Verification items for this drawing (mm, ordinates from the low corner). A direction names the side the tool comes from. Round coordinates to 2 decimals unless told otherwise and drop trailing zeros. Loops run counter-clockwise (first coordinate to the right, second up) from the corner with the lowest first, then second, coordinate; pieces in that order, holes last. Notation, with made-up numbers: M 35,67.25 L 66,67.25 A7 cw 66,75.25 Z; hole C 5,71 d9. An arc over 180 degrees is marked long. Write item = value, one per line. Start each with the question number.
(1) Cross-section at A-A on x = 21.5. Record the boundary of the cut face in (y, z), plus the area to 3 significant figures.
(2) Cross-section at D-D on x = 12. Record the boundary of the cut face in (y, z), plus the area to 3 significant figures.
(3) Mould release check, pull along Y, two halves, no side actions. Record for the marked faces 5, 6, 7 and 8: pulls with the +Y half, pulls with the -Y half, needs draft (parallel to the pull), parting line crosses it, or undercut.
(4) Set-up check for the marked faces 1, 2, 3 and 4: record each of +Z, -Z, +X, -X, +Y, -Y from which the full face is reachable in a straight line by a thin tool's end or side.
(5) Cross-section at B-B on y = 27.6. Record the boundary of the cut face in (x, z).
(6) Scan lines: L1, parallel to Y at x = 21.5, z = 6.5; L2, parallel to X at y = 27.5, z = 5; L3, parallel to Z at x = 8.5, y = 14.5. Record each from-to range of solid material in increasing order. Write a range as from..to.
(7) Cross-section at C-C on y = 5. Record the boundary of the cut face in (x, z).
(8) Go/stop test with flat-tipped pins: P1, Ø16, axis at x = 15.5, z = 21.5, coming from the +Y side; P2, Ø5, axis at y = 2.5, z = 14.5, coming from the -X side; P3, Ø11, axis at y = 5.5, z = 20.5, coming from the +X side. Record where each tip stops, or that it passes through.
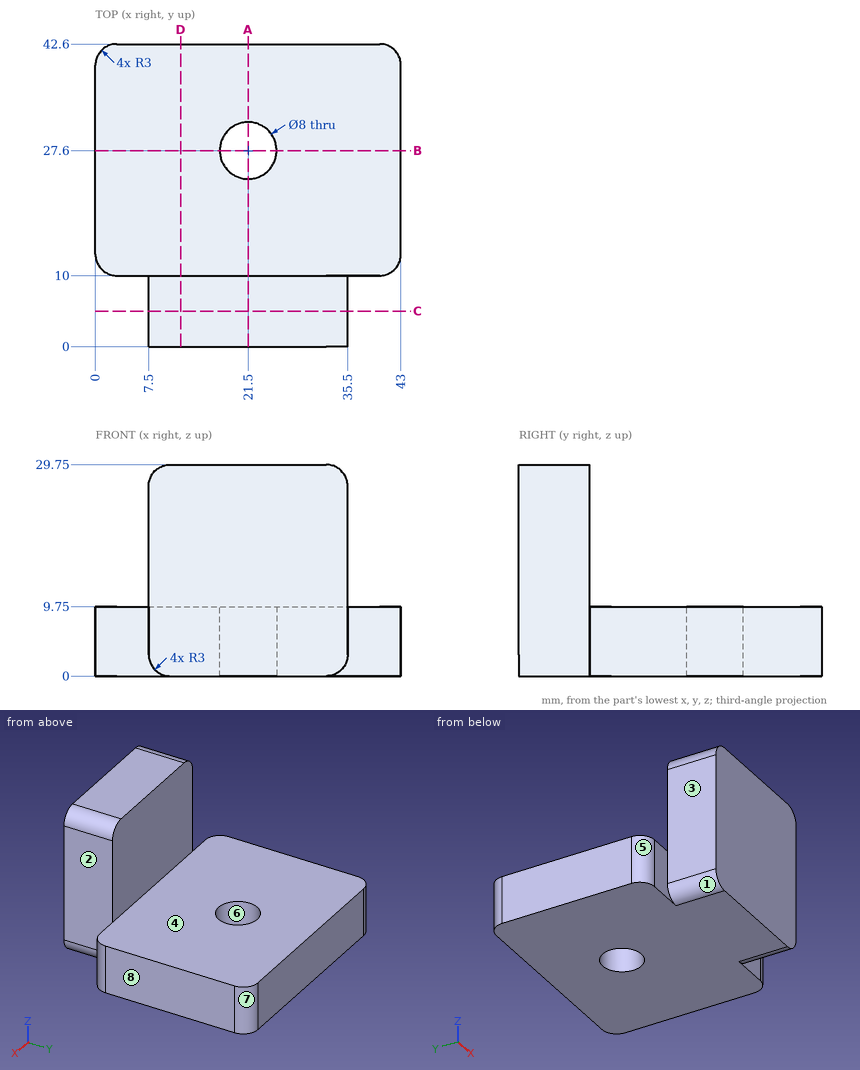
Result:
q1.outline = M 0,0 L 23.6,0 L 23.6,9.75 L 10,9.75 L 10,29.75 L 0,29.75 Z; M 31.6,0 L 42.6,0 L 42.6,9.75 L 31.6,9.75 Z
q1.area = 537 mm^2
q2.outline = M 0,0 L 42.6,0 L 42.6,9.75 L 10,9.75 L 10,29.75 L 0,29.75 Z
q2.area = 615 mm^2
q3.face_5 = pulls with the -Y half
q3.face_6 = undercut
q3.face_7 = pulls with the +Y half
q3.face_8 = needs draft
q4.face_1 = -Z, -X, -Y
q4.face_2 = +Z, -Z, +X, -Y
q4.face_3 = +Z, -Z, -X, -Y
q4.face_4 = +Z, +X, -X, +Y
q5.outline = M 0,0 L 17.5,0 L 17.5,9.75 L 0,9.75 Z; M 25.5,0 L 43,0 L 43,9.75 L 25.5,9.75 Z
q6.L1 = 0..23.6, 31.6..42.6
q6.L2 = 0..17.5, 25.5..43
q6.L3 = 0..9.75
q7.outline = M 7.5,3 A3 ccw 10.5,0 L 32.5,0 A3 ccw 35.5,3 L 35.5,26.75 A3 ccw 32.5,29.75 L 10.5,29.75 A3 ccw 7.5,26.75 Z
q8.P1 = 10
q8.P2 = 7.5
q8.P3 = 35.5
